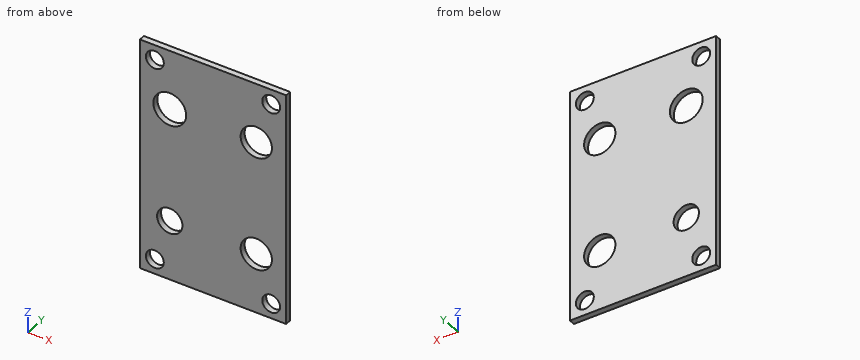
from build123d import *

# Parameters (mm, degrees)
CROQUIS1_W              = 49
CROQUIS1_H              = 73
CROQUIS1_R              = 5.25
CROQUIS1_R_2            = 5.5
CROQUIS1_R_3            = 4.25
CROQUIS1_R_4            = 3
SALIENTE_EXTRUIR4_DEPTH = 2
CROQUIS7_W              = 49
CROQUIS7_H              = 5
SALIENTE_EXTRUIR5_DEPTH = 2
CROQUIS8_R              = 3
CORTAR_EXTRUIR2_DEPTH   = 10


with BuildPart() as part:
    # Croquis1 → Saliente-Extruir4 (new body)
    with BuildSketch(Plane(origin=(0, 0, 0), x_dir=(1, 0, 0), z_dir=(0, 1, 0))):
        with Locations((0, 0.5)):
            Rectangle(CROQUIS1_W, CROQUIS1_H)
        with Locations(Location((14.5, -21.1, 0), (0, 0, 270))):
            Circle(CROQUIS1_R, mode=Mode.SUBTRACT)
        with Locations(Location((-14.5, -21.1, 0), (0, 0, 270))):
            Circle(CROQUIS1_R_2, mode=Mode.SUBTRACT)
        with Locations(Location((-14.5, 17, 0), (0, 0, 270))):
            Circle(CROQUIS1_R_3, mode=Mode.SUBTRACT)
        with Locations(Location((14.5, 17, 0), (0, 0, 270))):
            Circle(CROQUIS1_R, mode=Mode.SUBTRACT)
        with Locations(Location((-19.5, 32, 0), (0, 0, 270))):
            Circle(CROQUIS1_R_4, mode=Mode.SUBTRACT)
        with Locations(Location((19.5, 32, 0), (0, 0, 270))):
            Circle(CROQUIS1_R_4, mode=Mode.SUBTRACT)
    extrude(amount=SALIENTE_EXTRUIR4_DEPTH)

    # Croquis7 → Saliente-Extruir5 (add)
    with BuildSketch(Plane(origin=(0, 2, 0), x_dir=(1, 0, 0), z_dir=(0, 1, 0))):
        with Locations((0, -38.5)):
            Rectangle(CROQUIS7_W, CROQUIS7_H)
    extrude(amount=-SALIENTE_EXTRUIR5_DEPTH)

    # Croquis8 → Cortar-Extruir2 (cut)
    with BuildSketch(Plane(origin=(0, 2, 0), x_dir=(1, 0, 0), z_dir=(0, 1, 0))):
        with Locations(Location((-19.5, -36, 0), (0, 0, 270))):
            Circle(CROQUIS8_R)
        with Locations(Location((19.5, -36, 0), (0, 0, 270))):
            Circle(CROQUIS8_R)
    extrude(amount=-CORTAR_EXTRUIR2_DEPTH, mode=Mode.SUBTRACT)


solid = part.part
Verification items for the finished model (mm, model axes). Coordinates: 2 decimals unless noted, no trailing zeros. Order: outer loops, then holes, each group sorted by start corner. A loop starts at its lowest first (then second) coordinate and runs counter-clockwise, first axis right, second up. Notation, with made-up numbers: M 69,-9.5 L 76,-9.5 A12 ccw 76,8.5 Z; hole C 63.25,39.25 d6. An arc over 180 degrees is marked long. One line per item, written item: value. Start each with the question number.
Item 1: Sectioned sample at B-B (x = -14.5). Enter the section's corners in (y, z), then the cut area to 3 significant figures.
Item 2: Sectioned sample at C-C (y = 1.3). Count the separate pieces of the cut face and the enclosed holes in it, then the cut area to 3 significant figures.
Item 3: Scan lines: probe 1 along X at (y, z) = (0.75, -32); probe 2 along X at (y, z) = (1.4, 21.1); probe 3 along Z at (x, y) = (-13.5, 1.95). Record each from-to range of solid material in increasing order.
Item 4: Gauge pin test, flat ends, axial feed: pin 1 (5 mm diameter, centred on x = -14.5, z = -17, fed in from +Y); pin 2 (12.5 mm diameter, centred on x = -14.5, z = 21.1, fed in from -Y). Record the tip position at first contact, or that the pin passes through.
Item 5: Sectioned sample at A-A (z = -17). Enter the section's corners in (x, y).
Conclusion:
1. outline: M 0,-37 L 2,-37 L 2,-21.25 L 0,-21.25 Z; M 0,-12.75 L 2,-12.75 L 2,15.6 L 0,15.6 Z; M 0,26.6 L 2,26.6 L 2,41 L 0,41 Z
1. area: 117 mm^2
2. separate pieces: 1
2. enclosed holes: 8
2. area: 3,380 mm^2
3. probe 1: x = -24.5 to -22.5, -16.5 to 16.5, 22.5 to 24.5
3. probe 2: x = -24.5 to -20, -9 to 9.25, 19.75 to 24.5
3. probe 3: z = -37 to -21.13, -12.87 to 15.69, 26.51 to 41
4. pin 1: passes through
4. pin 2: stops at y = 0
5. outline: M -24.5,0 L -18.75,0 L -18.75,2 L -24.5,2 Z; M -10.25,0 L 9.25,0 L 9.25,2 L -10.25,2 Z; M 19.75,0 L 24.5,0 L 24.5,2 L 19.75,2 Z
